Geometry check sheet. Reference: the model listing, model coordinates, mm. A direction names the side the tool comes from. Coordinates: 2 decimals unless noted, no trailing zeros. Write each loop counter-clockwise with the first axis right and the second up, starting at its lowest first coordinate (ties: lowest second). Pieces come first, ordered by that corner, then holes. Notation, with made-up numbers: (54.5, -11.5) -> (113.5, -11.5) arc R30 cw to (113.5, 16.5) -> close; hole circle Ø5 at (13, 18.5). An arc over 180 degrees is marked (long way). Answer as CSV lines item,"result".
```python
from build123d import *

# Parameters (mm, degrees)
SKETCH1_R                 = 140
SKETCH1_R_2               = 134
BOSS_EXTRUDE1_DEPTH       = 184.7
M2X0_4_TAPPED_HOLE2_D     = 1.6
M2X0_4_TAPPED_HOLE2_DEPTH = 3.6
M2X0_4_TAPPED_HOLE2_TIP   = 0.480688495
SKETCH5_W                 = 12.9
SKETCH5_H                 = 57.15
CUT_EXTRUDE1_DEPTH        = 140


with BuildPart() as part:
    # Sketch1 → Boss-Extrude1 (new body)
    with BuildSketch(Plane.XY):
        Circle(SKETCH1_R)
        Circle(SKETCH1_R_2, mode=Mode.SUBTRACT)
    extrude(amount=BOSS_EXTRUDE1_DEPTH)

    # M2x0.4 Tapped Hole2
    with Locations(Plane(origin=(0, 0, 0), x_dir=(-1, 0, 0), z_dir=(0, 0, -1))):
        with Locations((0, 137), (137, 0), (93.955376533, 99.116205732), (96.874, -96.874), (0, -137), (-96.874, -96.874), (-137, 0), (-96.874, 96.874)):
            Hole(M2X0_4_TAPPED_HOLE2_D / 2, depth=M2X0_4_TAPPED_HOLE2_DEPTH)
            with Locations((0, 0, -(M2X0_4_TAPPED_HOLE2_DEPTH + M2X0_4_TAPPED_HOLE2_TIP / 2))):  # 118° drill point
                Cone(0, M2X0_4_TAPPED_HOLE2_D / 2, M2X0_4_TAPPED_HOLE2_TIP, mode=Mode.SUBTRACT)

    # Sketch5 → Cut-Extrude1 (cut)
    with BuildSketch(Plane(origin=(0, 0, 0), x_dir=(0, 0, -1), z_dir=(1, 0, 0))):
        with Locations((-129.25, 0)):
            Rectangle(SKETCH5_W, SKETCH5_H)
    extrude(amount=CUT_EXTRUDE1_DEPTH, mode=Mode.SUBTRACT)


solid = part.part
```
Item 1: Depth check by flat-ended pin: pin 1 Ø4 at (y, z) = (23.5, 49) entering from -X; pin 2 Ø6 at (y, z) = (105.5, 67) entering from -X; pin 3 Ø3 at (y, z) = (-64, 84.5) entering from -X; pin 4 Ø7.5 at (x, y) = (137, 2.5) entering from -Z. Enter the tip coordinate at first touch or a pass-through.
Responses:
pin 1,"stops at x = -138.34"
pin 2,"stops at x = -95.36"
pin 3,"stops at x = -125.27"
pin 4,"stops at z = 0"
Item 2: Set-up check for faces 1 (the cylindrical face through (-29.049, -130.814, 91.057)), 2 (the flat face through (136, 0, 135.7)): record each of +Z, -Z, +X, -X, +Y, -Y from which the full face is reachable in a straight line by a thin tool's end or side.
Responses:
face 1,"+Z, -Z"
face 2,"+X"
Item 3: Cross-section at C-C, the plane y = 86.5. Record the cut outline in (x, z).
Responses:
outline,"(-110.08, 0) -> (-102.34, 0) -> (-102.34, 184.7) -> (-110.08, 184.7) -> close; (102.34, 0) -> (110.08, 0) -> (110.08, 184.7) -> (102.34, 184.7) -> close"
Item 4: Cross-section at B-B, the plane y = -8.5. Record the cut outline in (x, z).
Responses:
outline,"(-139.74, 0) -> (-133.73, 0) -> (-133.73, 184.7) -> (-139.74, 184.7) -> close; (133.73, 0) -> (139.74, 0) -> (139.74, 122.8) -> (133.73, 122.8) -> close; (133.73, 135.7) -> (139.74, 135.7) -> (139.74, 184.7) -> (133.73, 184.7) -> close"
Item 5: Thickness scan on probe 1 along Y at (x, z) = (4, 87.5); probe 2 along Y at (x, z) = (76.5, 127); probe 3 along X at (y, z) = (117.5, 164.5). Record the ranges inside material, lowest first.
Responses:
probe 1,"y = -139.94 to -133.94, 133.94 to 139.94"
probe 2,"y = -117.25 to -110.02, 110.02 to 117.25"
probe 3,"x = -76.12 to -64.42, 64.42 to 76.12"
Item 6: Cross-section at D-D, the plane z = 110.5. Record the cut outline in (x, y), plus the area to 3 significant figures.
Responses:
outline,"circle Ø280 at (0, 0); hole circle Ø268 at (0, 0)"
area,"5,160 mm2"
Item 7: Cross-section at A-A, the plane x = 15.5. Record the cut outline in (y, z), plus the area to 3 significant figures.
Responses:
outline,"(-139.14, 0) -> (-133.1, 0) -> (-133.1, 184.7) -> (-139.14, 184.7) -> close; (133.1, 0) -> (139.14, 0) -> (139.14, 184.7) -> (133.1, 184.7) -> close"
area,"2,230 mm2"
Item 8: Release check for a two-part mould opening along Z. For faces 3 (the flat face through (136, 0, 122.8)), 4 (the flat face through (71.9, -113.4, 184.7)), 5 (the flat face through (71.9, -113.4, 0)) record: +Z half, -Z half, draft (parallel to the pull), parting line (faces both ways), or undercut.
Responses:
face 3,"undercut"
face 4,"+Z half"
face 5,"-Z half"
